from build123d import *

# Parameters (mm, degrees)
SKETCH3_R                = 5
SKETCH3_R_2              = 3.3
BOSS_EXTRUDE3_DEPTH      = 10
BOSS_EXTRUDE3_DEPTH_BACK = 5
SKETCH10_R               = 12.775
SKETCH10_R_2             = 3.65
BOSS_EXTRUDE5_DEPTH      = 2
SKETCH11_R               = 11.275
SKETCH11_R_2             = 6.775
BOSS_EXTRUDE6_DEPTH      = 0.8
SKETCH12_R               = 1.25
CUT_EXTRUDE2_DEPTH       = 2.75
FILLET3_R                = 1
SKETCH13_R               = 12.775
SKETCH13_R_2             = 11.275
BOSS_EXTRUDE7_DEPTH      = 10
SKETCH14_R               = 11.7
CUT_EXTRUDE3_DEPTH       = 9.2
CUT_EXTRUDE5_DEPTH       = 16
SKETCH16_R               = 4
CUT_EXTRUDE6_DEPTH       = 14


with BuildPart() as part:
    # Sketch3 → Boss-Extrude3 (new body, two sides)
    with BuildSketch(Plane(origin=(0, 0, 0), x_dir=(0, 0, -1), z_dir=(1, 0, 0))) as boss_extrude3_sk:
        Circle(SKETCH3_R)
        Circle(SKETCH3_R_2, mode=Mode.SUBTRACT)
    extrude(amount=BOSS_EXTRUDE3_DEPTH)
    extrude(boss_extrude3_sk.sketch, amount=-BOSS_EXTRUDE3_DEPTH_BACK)

    # Sketch10 → Boss-Extrude5 (add)
    with BuildSketch(Plane(origin=(10, 0, 0), x_dir=(0, 0, -1), z_dir=(1, 0, 0))):
        Circle(SKETCH10_R)
        Circle(SKETCH10_R_2, mode=Mode.SUBTRACT)
    extrude(amount=-BOSS_EXTRUDE5_DEPTH)

    # Sketch11 → Boss-Extrude6 (add)
    with BuildSketch(Plane(origin=(10, 0, 0), x_dir=(0, 0, -1), z_dir=(1, 0, 0))):
        Circle(SKETCH11_R)
        Circle(SKETCH11_R_2, mode=Mode.SUBTRACT)
    extrude(amount=BOSS_EXTRUDE6_DEPTH)

    # Sketch12 → Cut-Extrude2 (cut)
    with BuildSketch(Plane(origin=(10.8, 0, 0), x_dir=(0, 0, -1), z_dir=(1, 0, 0))):
        with BuildLine():
            ThreePointArc((9.330017017, -4.665), (8.705017017, -3.582468245), (7.455017017, -3.582468245))
            Line((7.455017017, -3.582468245), (8.080017017, -4.665))
            Line((8.080017017, -4.665), (6.830017017, -4.665))
            ThreePointArc((6.830017017, -4.665), (8.080017017, -5.915), (9.330017017, -4.665))
        make_face()
        with BuildLine():
            Line((8.080017017, -4.665), (7.455017017, -3.582468245))
            ThreePointArc((7.455017017, -3.582468245), (6.997485263, -4.04), (6.830017017, -4.665))
            Line((6.830017017, -4.665), (8.080017017, -4.665))
        make_face()
        with BuildLine():
            Line((0.625, 8.247468245), (0, 9.33))
            Line((0, 9.33), (-0.625, 8.247468245))
            ThreePointArc((-0.625, 8.247468245), (0, 8.08), (0.625, 8.247468245))
        make_face()
        with BuildLine():
            Line((-0.625, 8.247468245), (0, 9.33))
            Line((0, 9.33), (0.625, 8.247468245))
            ThreePointArc((0.625, 8.247468245), (1.082531755, 8.705), (1.25, 9.33))
            ThreePointArc((1.25, 9.33), (-0.625, 10.412531755), (-0.625, 8.247468245))
        make_face()
        with Locations((-8.080017017, -4.665)):
            Circle(SKETCH12_R)
    extrude(amount=-CUT_EXTRUDE2_DEPTH, mode=Mode.SUBTRACT)

    # Fillet3
    fillet3_edges = [part.edges().sort_by_distance(p)[0] for p in [
        (8, 0, 12.775),
    ]]
    fillet(fillet3_edges, radius=FILLET3_R)

    # Sketch13 → Boss-Extrude7 (add)
    with BuildSketch(Plane(origin=(10, 0, 0), x_dir=(0, 0, -1), z_dir=(1, 0, 0))):
        Circle(SKETCH13_R)
        Circle(SKETCH13_R_2, mode=Mode.SUBTRACT)
    extrude(amount=BOSS_EXTRUDE7_DEPTH)

    # Sketch14 → Cut-Extrude3 (cut)
    with BuildSketch(Plane(origin=(20, 0, 0), x_dir=(0, 0, -1), z_dir=(1, 0, 0))):
        Circle(SKETCH14_R)
    extrude(amount=-CUT_EXTRUDE3_DEPTH, mode=Mode.SUBTRACT)

    # Sketch15 → Cut-Extrude5 (cut)
    with BuildSketch(Plane(origin=(0, 0, 0), x_dir=(1, 0, 0), z_dir=(0, 1, 0))):
        with BuildLine():
            Line((15.430071931, 3.675), (20, 3.675))
            Line((20, 3.675), (20, 11.775))
            Line((20, 11.775), (15.430071931, 11.775))
            ThreePointArc((15.430071931, 11.775), (11.380071931, 7.725), (15.430071931, 3.675))
        make_face()
    extrude(amount=CUT_EXTRUDE5_DEPTH, mode=Mode.SUBTRACT)

    # Sketch16 → Cut-Extrude6 (cut)
    with BuildSketch(Plane.ZY.offset(5)):
        Circle(SKETCH16_R)
    extrude(amount=-CUT_EXTRUDE6_DEPTH, mode=Mode.SUBTRACT)


solid = part.part
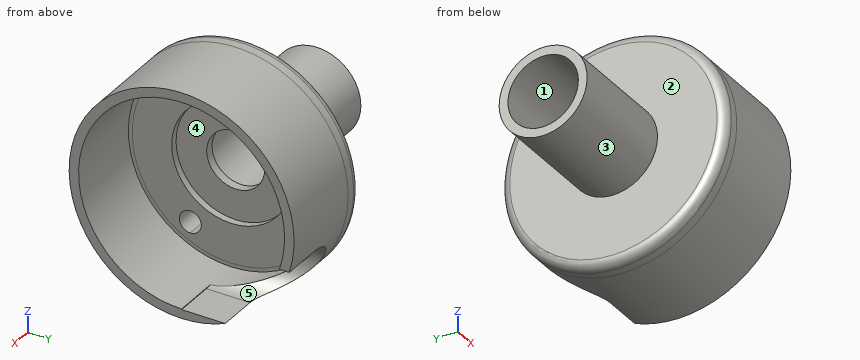
Geometry check sheet. Reference: the model listing, model coordinates, mm. Face numbers are marked on the shaded views. A direction names the side the tool comes from. Give positions to 0.01 mm unless a question says otherwise; leave off trailing zeros. Order: outer loops, then holes, each group sorted by start corner. A loop starts at its lowest first (then second) coordinate and runs counter-clockwise, first axis right, second up. Notation, with made-up numbers: M -40,63 L -28,63 A13 cw -28,82 Z; hole C -22,-11.75 d9. An arc over 180 degrees is marked long. Use a Markdown table: item, result.
Item 1: Material ranges on line 1 along Y through (x, z) = (13.75, 0) (3 decimals); line 2 along X through (y, z) = (2, 3.75); line 3 along X through (y, z) = (5.25, -7.25), recorded low to high.
Answers follow:
| item | result |
|---|---|
| line 1 | y = -12.775 to -11.7, 11.7 to 12.775 |
| line 2 | x = -5 to 10 |
| line 3 | x = 8 to 10.8 |
Item 2: Section check B-B (x = -0.5). Record the cut outline in (y, z).
Answers follow:
| item | result |
|---|---|
| outline | C 0,0 d10; hole C 0,0 d8 |
Item 3: Draft check along Z on the marked faces 1, 2 and 3. Enter one of: +Z half, -Z half, draft (parallel to the pull), parting line (faces both ways), or undercut.
Answers follow:
| item | result |
|---|---|
| face 1 | undercut |
| face 2 | draft |
| face 3 | parting line |
Item 4: Depth check by flat-ended pin: P1, Ø4, axis at x = 9, y = -7.5, coming from the +Z side; P2, Ø9, axis at y = 0, z = 0, coming from the +X side; P3, Ø1.5, axis at y = 9.5, z = -8.5, coming from the +X side. Enter the tip coordinate at first touch or a pass-through.
Answers follow:
| item | result |
|---|---|
| P1 | stops at z = 11.53 |
| P2 | stops at x = 10 |
| P3 | stops at x = 11.61 |
Item 5: Tool access check on the marked faces 4 and 5. Record the directions out of +Z, -Z, +X, -X, +Y, -Y that give a thin tool (end or side, any length) a straight path to the whole face; none if there is none.
Answers follow:
| item | result |
|---|---|
| face 4 | +X |
| face 5 | +X, +Y |
